Autodesk Inventor part; units mm, degrees
ref_plane "YZ Plane" through (0, 0, 0) normal (1, 0, 0) x (0, 1, 0)
ref_plane "XZ Plane" through (0, 0, 0) normal (0, 1, 0) x (-1, 0, 0)
ref_plane "XY Plane" through (0, 0, 0) normal (0, 0, 1) x (1, 0, 0)
sketch "Sketch1" plane through (0, 0, 0) normal (0, 0, 1) x (1, 0, 0)
  line L0 (-11.9064, 7.7279) -> (8.0936, 7.7279)
  line L1 (8.0936, 7.7279) -> (8.0936, -12.2721)
  line L2 (8.0936, -12.2721) -> (-11.9064, -12.2721)
  line L3 (-11.9064, -12.2721) -> (-11.9064, 7.7279)
  point P0 (0, 0)
  dimension "d0" = 20
  dimension "d1" = 20
extrude "Extrusion1" add sketch "Sketch1" along normal blind 250
sketch "Sketch2" plane through (0, 0, 250) normal (0, 0, 1) x (1, 0, 0)
  circle A0 centre (-1.9064, -2.2721) radius 2
  line L0 (-11.9064, -12.2721) -> (8.0936, -12.2721)
  line L1 (8.0936, -12.2721) -> (8.0936, 7.7279)
  point P0 (0, 0)
  dimension "d4" = 4
  dimension "d5" = 10
  dimension "d6" = 10
extrude "Extrusion2" cut sketch "Sketch2" against normal blind 250
properties part number "2020x260mm" material "ABS Plastic"
Can you work these out from the model? Positions are in its coordinate system, mm. Round coordinates to 2 decimals unless told otherwise and drop trailing zeros. Loops run counter-clockwise (first coordinate to the right, second up) from the corner with the lowest first, then second, coordinate; pieces in that order, holes last.
Item 1: Please list where these lines run through material, in increasing order: L1, parallel to Y at x = -1.5, z = 11.5; L2, parallel to X at y = -3.25, z = 179.5; L3, parallel to X at y = -3.5, z = 92.
Item 2: Suppose I cut it at A-A, the plane z = 44. Write out the boundary of the cut face in (x, y), then the cut area to 3 significant figures.
Item 3: Will this pin go through, and if not, where does the flat tip stop? pin 1 Ø3.5 at (x, y) = (-1.91, -2.27) entering from -Z.
Item 4: If we mould it in two halves opening along X, with no side actions, what happens to faces 1 (the flat face through (-2, 0, 0)), 2 (the flat face through (8.094, -2, 123)), 3 (the flat face through (-11.906, -2, 123)), 4 (the cylindrical face through (-0.06, -3.04, 126.75))? For each: +X half, -X half, draft (parallel to the pull), parting line (faces both ways), or undercut.
Reported:
1. L1: y = -12.27 to -4.23, -0.31 to 7.73
1. L2: x = -11.91 to -3.65, -0.16 to 8.09
1. L3: x = -11.91 to -3.49, -0.33 to 8.09
2. outline: (-11.91, -12.27) - (8.09, -12.27) - (8.09, 7.73) - (-11.91, 7.73) - close; hole circle Ø4 at (-1.91, -2.27)
2. area: 387 mm2
3. pin 1: passes through
4. face 1: draft
4. face 2: +X half
4. face 3: -X half
4. face 4: undercut
